Here's the drawing with two shaded views (mm, measured from the low corner). I have some questions. A direction names the side the tool comes from. Coordinates: 2 decimals unless noted, no trailing zeros. Order: outer loops, then holes, each group sorted by start corner. A loop starts at its lowest first (then second) coordinate and runs counter-clockwise, first axis right, second up. Notation, with made-up numbers: (24, 16.5) -> (37, 16.5) arc R18 ccw to (37, 38.5) -> close; hole circle Ø6 at (-4.75, 20.5). An arc over 180 degrees is marked (long way). Answer as a JSON object with one key per item and string values. Group by question number.
(1) I want a section at C-C, the plane y = 29. List the corners of the cut face in (x, z) for me.
(2) For pin 1 (1 mm diameter, centred on y = 18, z = 10.5, fed in from +X), with a flat end and sliding along its axis, tell me the tip position at first contact or that it passes through.
(3) I need wall thicknesses on line 1 (Z direction, x = 25.4, y = 6.5); line 2 (Y direction, x = 25.4, z = 22); line 3 (X direction, y = 3, z = 41). Which ranges of each line are inside material? Lowest first, please.
(4) Which directions (+Z, -Z, +X, -X, +Y, -Y) give clear straight access to the entire face, cutting with the end or side of a thin tool? Please do the marked faces 1 and 2.
(5) I want a section at D-D, the plane x = 16. List the corners of the cut face in (y, z) for me.
(6) I want a section at A-A, the plane x = 25.4. List the corners of the cut face in (y, z) for me.
(7) I want a section at B-B, the plane z = 43. List the corners of the cut face in (x, y) for me.
(8) If we mould it in two halves opening along X, with no side actions, what happens to the marked faces 3, 4, 5 and 6? For each: pulls with the +X half, pulls with the -X half, needs draft (parallel to the pull), parting line crosses it, or undercut.
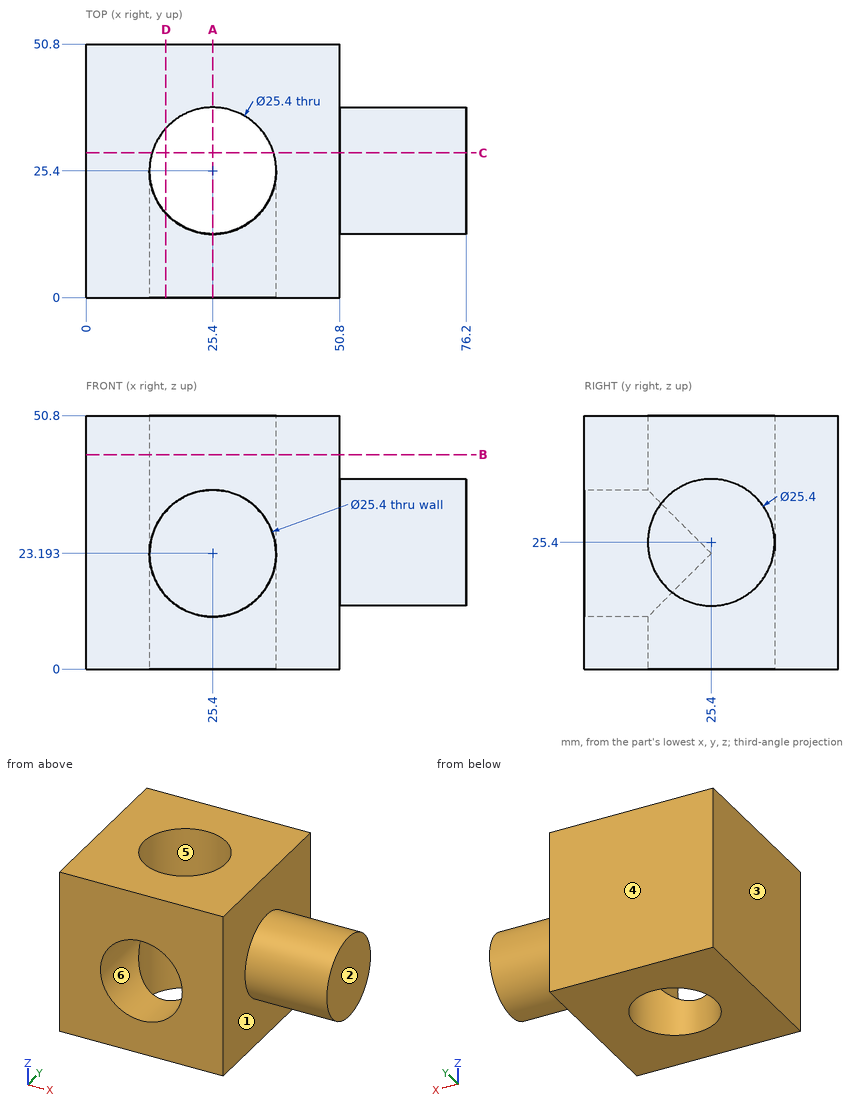
Computed values:
{
 "1": {"outline": "(0, 0) -> (13.22, 0) -> (13.22, 50.8) -> (0, 50.8) -> close; (37.58, 0) -> (50.8, 0) -> (50.8, 13.22) -> (76.2, 13.22) -> (76.2, 37.58) -> (50.8, 37.58) -> (50.8, 50.8) -> (37.58, 50.8) -> close"},
 "2": {"pin 1": "stops at x = 50.8"},
 "3": {"line 1": "z = 0 to 10.49, 35.89 to 50.8", "line 2": "y = 38.1 to 50.8", "line 3": "x = 0 to 50.8"},
 "4": {"face 1": "+X", "face 2": "+Z, -Z, +X, +Y, -Y"},
 "5": {"outline": "(0, 0) -> (16.86, 0) -> (16.86, 14.65) -> (0, 14.65) -> close; (0, 31.73) -> (16.86, 31.73) -> (16.86, 50.8) -> (0, 50.8) -> close; (33.94, 0) -> (50.8, 0) -> (50.8, 50.8) -> (33.94, 50.8) -> close"},
 "6": {"outline": "(0, 0) -> (12.7, 0) -> (12.7, 10.49) -> (0, 10.49) -> close; (0, 35.89) -> (12.7, 35.89) -> (12.7, 50.8) -> (0, 50.8) -> close; (38.1, 0) -> (50.8, 0) -> (50.8, 50.8) -> (38.1, 50.8) -> close"},
 "7": {"outline": "(0, 0) -> (50.8, 0) -> (50.8, 50.8) -> (0, 50.8) -> close; hole circle Ø25.4 at (25.4, 25.4)"},
 "8": {"face 3": "pulls with the -X half", "face 4": "needs draft", "face 5": "undercut", "face 6": "undercut"}
}
